from build123d import *

# Parameters (mm, degrees)
ESBO_O1_W                = 90
ESBO_O1_H                = 93
RESSALTO_EXTRUS_O1_DEPTH = 9.53
ESBO_O3_R                = 32.51
CORTE_EXTRUS_O2_DEPTH    = 5
ESBO_O2_R                = 2.6
CORTE_EXTRUS_O1_DEPTH    = 19
CORTE_EXTRUS_O3_REACH    = 66.902
ESBO_O4_R                = 27.5
CORTE_EXTRUS_O4_REACH    = 67.407
ESBO_O5_W                = 27.5
ESBO_O5_H                = 13
CORTE_EXTRUS_O5_REACH    = 67.407
ESBO_O6_W                = 6
ESBO_O6_H                = 26.167415493
CORTE_EXTRUS_O6_REACH    = 80.481
ESBO_O7_R                = 2.5


with BuildPart() as part:
    # Esboço1 → Ressalto-extrusão1 (new body)
    with BuildSketch(Plane(origin=(0, 0, 0), x_dir=(1, 0, 0), z_dir=(0, 1, 0))):
        Rectangle(ESBO_O1_W, ESBO_O1_H)
    extrude(amount=RESSALTO_EXTRUS_O1_DEPTH)

    # Esboço3 → Corte-extrusão2 (cut)
    with BuildSketch(Plane(origin=(0, 9.53, 0), x_dir=(1, 0, 0), z_dir=(0, 1, 0))):
        with Locations(Location((0, 3.5, 0), (0, 0, 270))):
            Circle(ESBO_O3_R)
    extrude(amount=-CORTE_EXTRUS_O2_DEPTH, mode=Mode.SUBTRACT)

    # Esboço2 → Corte-extrusão1 (cut)
    with BuildSketch(Plane(origin=(0, 0, -46.5), x_dir=(-1, 0, 0), z_dir=(0, 0, -1))):
        with Locations((-40, 4.765)):
            Circle(ESBO_O2_R)
        with Locations((-25, 4.765)):
            Circle(ESBO_O2_R)
        with Locations((25, 4.76)):
            Circle(ESBO_O2_R)
        with Locations((40, 4.765)):
            Circle(ESBO_O2_R)
    extrude(amount=-CORTE_EXTRUS_O1_DEPTH, mode=Mode.SUBTRACT)

    # Esboço4 → Corte-extrusão3 (cut, up to next)
    with BuildSketch(Plane(origin=(0, 4.53, 0), x_dir=(1, 0, 0), z_dir=(0, 1, 0)), mode=Mode.PRIVATE) as corte_extrus_o3_sk1:
        with Locations(Location((0, 3.5, 0), (0, 0, 270))):
            Circle(ESBO_O4_R)
    corte_extrus_o3_tool1 = extrude(corte_extrus_o3_sk1.sketch, amount=-CORTE_EXTRUS_O3_REACH, mode=Mode.PRIVATE) & part.part
    add(corte_extrus_o3_tool1.solids().sort_by_distance((0, 4.53, -3.5))[0], mode=Mode.SUBTRACT)

    # Esboço5 → Corte-extrusão4 (cut, up to next)
    with BuildSketch(Plane(origin=(0, 9.53, 0), x_dir=(1, 0, 0), z_dir=(0, 1, 0)), mode=Mode.PRIVATE) as corte_extrus_o4_sk1:
        with Locations((31.25, -40)):
            Rectangle(ESBO_O5_W, ESBO_O5_H)
    corte_extrus_o4_tool1 = extrude(corte_extrus_o4_sk1.sketch, amount=-CORTE_EXTRUS_O4_REACH, mode=Mode.PRIVATE) & part.part
    # Esboço5 → Corte-extrusão4 (cut, up to next)
    with BuildSketch(Plane(origin=(0, 9.53, 0), x_dir=(1, 0, 0), z_dir=(0, 1, 0)), mode=Mode.PRIVATE) as corte_extrus_o4_sk2:
        with Locations((-31.25, -40)):
            Rectangle(ESBO_O5_W, ESBO_O5_H)
    corte_extrus_o4_tool2 = extrude(corte_extrus_o4_sk2.sketch, amount=-CORTE_EXTRUS_O4_REACH, mode=Mode.PRIVATE) & part.part
    add(corte_extrus_o4_tool1.solids().sort_by_distance((31.25, 9.53, 40))[0], mode=Mode.SUBTRACT)
    add(corte_extrus_o4_tool2.solids().sort_by_distance((-31.25, 9.53, 40))[0], mode=Mode.SUBTRACT)

    # Esboço6 → Corte-extrusão5 (cut, up to next)
    with BuildSketch(Plane(origin=(0, 9.53, 0), x_dir=(1, 0, 0), z_dir=(0, 1, 0)), mode=Mode.PRIVATE) as corte_extrus_o5_sk1:
        with Locations((0, -33.416292254)):
            Rectangle(ESBO_O6_W, ESBO_O6_H)
    corte_extrus_o5_tool1 = extrude(corte_extrus_o5_sk1.sketch, amount=-CORTE_EXTRUS_O5_REACH, mode=Mode.PRIVATE) & part.part
    add(corte_extrus_o5_tool1.solids().sort_by_distance((0, 9.53, 33.416292))[0], mode=Mode.SUBTRACT)

    # Corte-extrusão6: up to this face of the body (flat: up to its plane)
    corte_extrus_o6_end = Plane(part.part.faces().sort_by_distance((17.5, 4.765, 40))[0])
    # Esboço7 → Corte-extrusão6 (cut, up to the picked face)
    with BuildSketch(Plane.ZY.offset(17.5), mode=Mode.PRIVATE) as corte_extrus_o6_sk1:
        with Locations((41.5, 4.765)):
            Circle(ESBO_O7_R)
    corte_extrus_o6_tool1 = split(extrude(corte_extrus_o6_sk1.sketch, amount=-CORTE_EXTRUS_O6_REACH, mode=Mode.PRIVATE), bisect_by=corte_extrus_o6_end, keep=Keep.BOTH, mode=Mode.PRIVATE)
    add(corte_extrus_o6_tool1.solids().sort_by(Axis((-17.5, 4.765, 41.5), (1, 0, 0)))[0], mode=Mode.SUBTRACT)


solid = part.part
For this review, take the finished solid that the model builds, in its own axes (mm). A direction names the side the tool comes from. Round coordinates to 2 decimals unless told otherwise and drop trailing zeros. Loops run counter-clockwise (first coordinate to the right, second up) from the corner with the lowest first, then second, coordinate; pieces in that order, holes last. Notation, with made-up numbers: (74.5, -7.75) - (102.5, -7.75) arc R28 cw to (102.5, 20.25) - close; hole circle Ø7 at (46, -5.75). An arc over 180 degrees is marked (long way). One line per item, written item: value. Start each with the question number.
Item 1: Take a section at C-C (x = -25). Give the boundary of the cut face in (y, z), plus the area to 3 significant figures.
Item 2: The part is to be moulded in two halves that separate along Z. For faces 6 (the flat face through (-25, 5, -27.5)), 7 (the flat face through (31, 5, 33.5)), 8 (the cylindrical face through (1.167, 2.297, -30.975)), say which applies: +Z half, -Z half, draft (parallel to the pull), parting line (faces both ways), or undercut.
Item 3: For faces 1 (the flat face through (17.5, 4.8, 38.6)), 2 (the flat face through (-31, 5, 33.5)), 3 (the flat face through (7.4, 4.53, -30.2)), 4 (the cylindrical face through (42.597, 4.879, -37.133)), 5 (the cylindrical face through (10.15, 3.81, 43.81)), list the 3-axis set-ups (+Z, -Z, +X, -X, +Y, -Y) from which the entire face can be reached by the end or side of a thin tool; tool diameter is ignored.
Item 4: Take a section at B-B (z = 9). Give the boundary of the cut face in (x, y).
Item 5: Take a section at A-A (x = -10.5). Give the boundary of the cut face in (y, z) (3 decimals), plus the area to 3 significant figures.
Item 6: Clearance check with flat-ended pins moving along their axes: pin 1 Ø5 at (x, y) = (25, 7) entering from +Z; pin 2 Ø1.6 at (x, y) = (41, 5.5) entering from -Z. State where each tip first meets the part, or that it passes through.
Item 7: Take a section at D-D (x = 40). Give the boundary of the cut face in (y, z) (3 decimals), plus the area to 3 significant figures.
Item 8: For L1, parallel to X at y = 8.45, z = -3.5; L2, parallel to Y at x = 40, z = -42 (3 decimals); L3, parallel to Y at x = -7.5, z = 41.5 (3 decimals), list the stretches that pass through material, from the lowest coordinate up.
Answer below:
1. outline: (0, -46.5) - (2.16, -46.5) - (2.16, -27.5) - (7.36, -27.5) - (7.36, -46.5) - (9.53, -46.5) - (9.53, -24.28) - (4.53, -24.28) - (4.53, -14.96) - (0, -14.96) - close; (0, 7.96) - (4.53, 7.96) - (4.53, 17.28) - (9.53, 17.28) - (9.53, 33.5) - (0, 33.5) - close
1. area: 352 mm2
2. face 6: -Z half
2. face 7: +Z half
2. face 8: undercut
3. face 1: +Z, +X, +Y, -Y
3. face 2: +Z, -X, +Y, -Y
3. face 3: +Y
3. face 4: -Z
3. face 5: +X, -X
4. outline: (-45, 0) - (-24.49, 0) - (-24.49, 4.53) - (-30.01, 4.53) - (-30.01, 9.53) - (-45, 9.53) - close; (24.49, 0) - (45, 0) - (45, 9.53) - (30.01, 9.53) - (30.01, 4.53) - (24.49, 4.53) - close
5. outline: (0, -46.5) - (9.53, -46.5) - (9.53, -34.268) - (4.53, -34.268) - (4.53, -28.917) - (0, -28.917) - close; (0, 21.917) - (4.53, 21.917) - (4.53, 27.268) - (9.53, 27.268) - (9.53, 46.5) - (0, 46.5) - close; hole circle Ø5 at (4.765, 41.5)
5. area: 329 mm2
6. pin 1: stops at z = 33.5
6. pin 2: stops at z = -27.5
7. outline: (0, -46.5) - (2.165, -46.5) - (2.165, -27.5) - (7.365, -27.5) - (7.365, -46.5) - (9.53, -46.5) - (9.53, 33.5) - (0, 33.5) - close
7. area: 664 mm2
8. L1: x = -45 to -32.51, 32.51 to 45
8. L2: y = 0 to 2.165, 7.365 to 9.53
8. L3: y = 0 to 2.265, 7.265 to 9.53
